The listing builds one solid part. Answer for the finished solid, in the listing's coordinates (mm). Coordinates: 2 decimals unless noted, no trailing zeros. Order: outer loops, then holes, each group sorted by start corner. A loop starts at its lowest first (then second) coordinate and runs counter-clockwise, first axis right, second up. Notation, with made-up numbers: (74.25, 89) - (84.25, 89) arc R16 cw to (84.25, 93) - close; hole circle Ø8 at (11.5, 66). An arc over 180 degrees is marked (long way). Use one line per item in the form item = value. Start each with the question number.
Item 1: Consider line 1 along Y through (x, z) = (-19, 22.5); line 2 along Y through (x, z) = (-3, 13.25). Determine where each line is inside the solid, lowest interval first. Write a range as [from, to].
Item 2: Section C-C, the plane x = -17.5 is taken. Write down the section's boundary in (y, z), and give its area (3 significant figures).
Item 3: Each of these flat-tipped pins is pushed along its axis until it touches: pin 1 Ø2 at (x, z) = (13.5, 16.5) entering from -Y; pin 2 Ø10 at (x, z) = (-8, 23.5) entering from -Y; pin 3 Ø2 at (x, z) = (11.5, 19) entering from -Y. Where does it stop, or does it pass through?
Item 4: Section A-A, the plane z = 13.5 is taken. Write down the section's boundary in (x, y), and give its area (3 significant figures).
Item 5: Section B-B, the plane x = -11 is taken. Write down the section's boundary in (y, z).
from build123d import *

# Parameters (mm, degrees)
BOSS_EXTRUDE1_DEPTH = 30


with BuildPart() as part:
    # Sketch1 → Boss-Extrude1 (new body)
    with BuildSketch(Plane.XY):
        with BuildLine():
            Line((0, 271.108554652), (-2.5, 271.108554652))
            Line((-2.5, 271.108554652), (-20.776742097, 264.45636455))
            Line((-20.776742097, 264.45636455), (-20.776742097, 221.692084557))
            Line((-20.776742097, 221.692084557), (-2.07767421, 218.394934374))
            Line((-2.07767421, 218.394934374), (0, 218.394934374))
            add(Edge.make_bspline(
                [(0, 218.394934374), (0, 235.966141134), (0, 253.537347893), (0, 271.108554652)],
                knots=[0.805688603, 0.805688603, 0.805688603, 0.805688603, 1, 1, 1, 1], degree=3))
        make_face()
        with BuildLine():
            Line((2.5, 271.108554652), (0, 271.108554652))
            add(Edge.make_bspline(
                [(0, 218.394934374), (0, 235.966141134), (0, 253.537347893), (0, 271.108554652)],
                knots=[0.805688603, 0.805688603, 0.805688603, 0.805688603, 1, 1, 1, 1], degree=3))
            Line((0, 218.394934374), (2.07767421, 218.394934374))
            Line((2.07767421, 218.394934374), (20.776742097, 221.692084557))
            Line((20.776742097, 221.692084557), (20.776742097, 264.45636455))
            Line((20.776742097, 264.45636455), (2.5, 271.108554652))
        make_face()
    extrude(amount=BOSS_EXTRUDE1_DEPTH)


solid = part.part
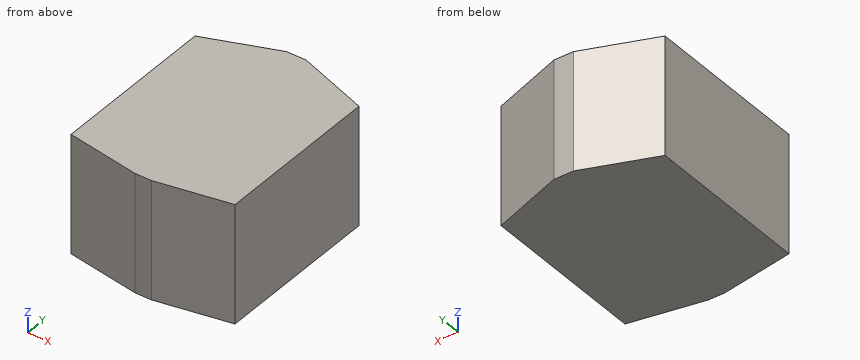
Response:
q1.line_1 = [221.38, 265.1]
q1.line_2 = [218.56, 270.93]
q2.outline = (221.11, 0) - (265.65, 0) - (265.65, 30) - (221.11, 30) - close
q2.area = 1,340 mm2
q3.pin_1 = 220.23
q3.pin_2 = 218.56
q3.pin_3 = 219.88
q4.outline = (-20.78, 221.69) - (-2.08, 218.39) - (2.08, 218.39) - (20.78, 221.69) - (20.78, 264.46) - (2.5, 271.11) - (-2.5, 271.11) - (-20.78, 264.46) - close
q4.area = 2,010 mm2
q5.outline = (219.97, 0) - (268.01, 0) - (268.01, 30) - (219.97, 30) - close
